Geometry check sheet. Reference: drawing and pictorial views, mm from the part's lowest x, y, z. A direction names the side the tool comes from. Round coordinates to 2 decimals unless told otherwise and drop trailing zeros. Order: outer loops, then holes, each group sorted by start corner. A loop starts at its lowest first (then second) coordinate and runs counter-clockwise, first axis right, second up.
(1) Draft check along X on the marked faces 3, 4 and 5. Enter one of: pulls with the +X half, pulls with the -X half, needs draft (parallel to the pull), parting line crosses it, or undercut.
(2) Gauge pin test, flat ends, axial feed: P1, Ø4, axis at x = 2, z = 10, coming from the +Y side; P2, Ø2, axis at y = 1.5, z = 4.5, coming from the -X side; P3, Ø2, axis at y = 4, z = 14.5, coming from the +X side; P4, Ø4, axis at y = 6, z = 9, coming from the +X side. Record the tip position at first contact, or that the pin passes through.
(3) Set-up check for the marked faces 1 and 2: record each of +Z, -Z, +X, -X, +Y, -Y from which the full face is reachable in a straight line by a thin tool's end or side.
(4) Cross-section at A-A on x = 5.25. Enter the section's corners in (y, z).
(5) Cross-section at B-B on y = 4.5. Enter the section's corners in (x, z).
(6) Thickness scan on L1, parallel to Y at x = 5.25, z = 4.5; L2, parallel to Z at x = 4.75, y = 4 (1 decimal); L3, parallel to X at y = 2.25, z = 2.75. Record the ranges inside material, lowest first.
(7) Cross-section at C-C on z = 8. Enter the section's corners in (x, y), and give its area (3 significant figures).
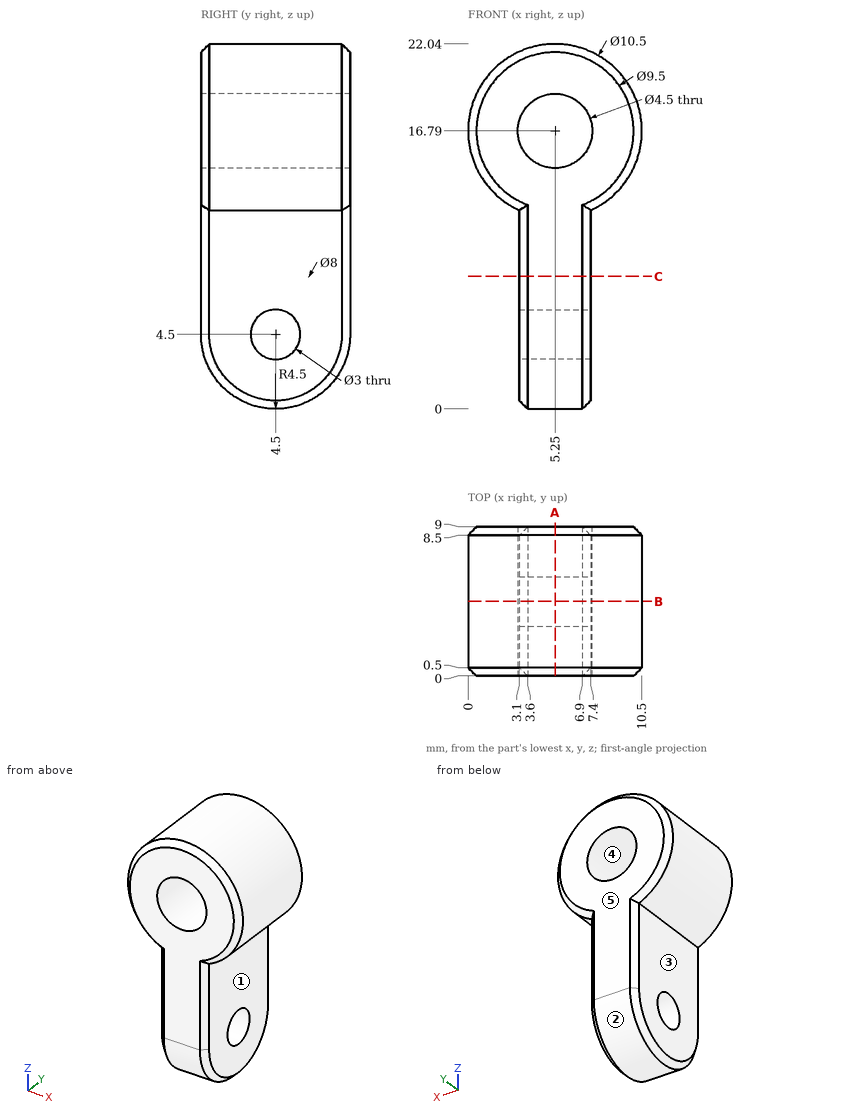
Found:
1. face 3: pulls with the -X half
1. face 4: undercut
1. face 5: needs draft
2. P1: stops at y = 9
2. P2: stops at x = 3.1
2. P3: stops at x = 10.34
2. P4: stops at x = 7.4
3. face 1: -Z, +X, +Y, -Y
3. face 2: -Z, +X, -X
4. outline: (0, 4.5) arc R4.5 ccw to (9, 4.5) - (9, 14.54) - (0, 14.54) - close; (0, 19.04) - (9, 19.04) - (9, 21.54) - (8.5, 22.04) - (0.5, 22.04) - (0, 21.54) - close; hole circle Ø3 at (4.5, 4.5)
5. outline: (3.1, 0.5) - (3.6, 0) - (6.9, 0) - (7.4, 0.5) - (7.4, 3) - (3.1, 3) - close; (3.1, 6) - (7.4, 6) - (7.4, 12) arc R5.25 ccw (long way) to (3.1, 12) - close; hole circle Ø4.5 at (5.25, 16.79)
6. L1: y = 0 to 3, 6 to 9
6. L2: z = 0 to 3.1, 5.9 to 14.6, 19 to 22
6. L3: x = 3.1 to 7.4
7. outline: (3.1, 0.5) - (3.6, 0) - (6.9, 0) - (7.4, 0.5) - (7.4, 8.5) - (6.9, 9) - (3.6, 9) - (3.1, 8.5) - close
7. area: 38.2 mm2
